Geometry check sheet. Reference: drawing and pictorial views, mm from the part's lowest x, y, z. Round coordinates to 2 decimals unless told otherwise and drop trailing zeros. Loops run counter-clockwise (first coordinate to the right, second up) from the corner with the lowest first, then second, coordinate; pieces in that order, holes last. Notation, with made-up numbers: (-39.5, 17.25) - (8.5, 17.25) arc R14 cw to (8.5, 39.25) - close; hole circle Ø7 at (-35, 8.5). An arc over 180 degrees is marked (long way). Put each result on its own line as item: value. Start each with the question number.
Item 1: Section check B-B, the plane x = 25. Record the cut outline in (y, z).
Item 2: Gauge pin test, flat ends, axial feed: pin 1 Ø5 at (x, y) = (153.5, 10.5) entering from -Z; pin 2 Ø4 at (x, z) = (25, 10) entering from +Y; pin 3 Ø2 at (x, z) = (25, 10) entering from +Y; pin 4 Ø4 at (x, z) = (159, 12) entering from +Y. Record the tip position at first contact, or that the pin passes through.
Item 3: Material ranges on line 1 along X through (y, z) = (2.15, 10); line 2 along Z through (x, y) = (25, 4.2); line 3 along Z through (x, y) = (77.5, 7.5), recorded low to high.
Item 4: Section check C-C, the plane x = 162. Record the cut outline in (y, z).
Item 5: Section check A-A, the plane y = 11.5. Record the cut outline in (x, z).
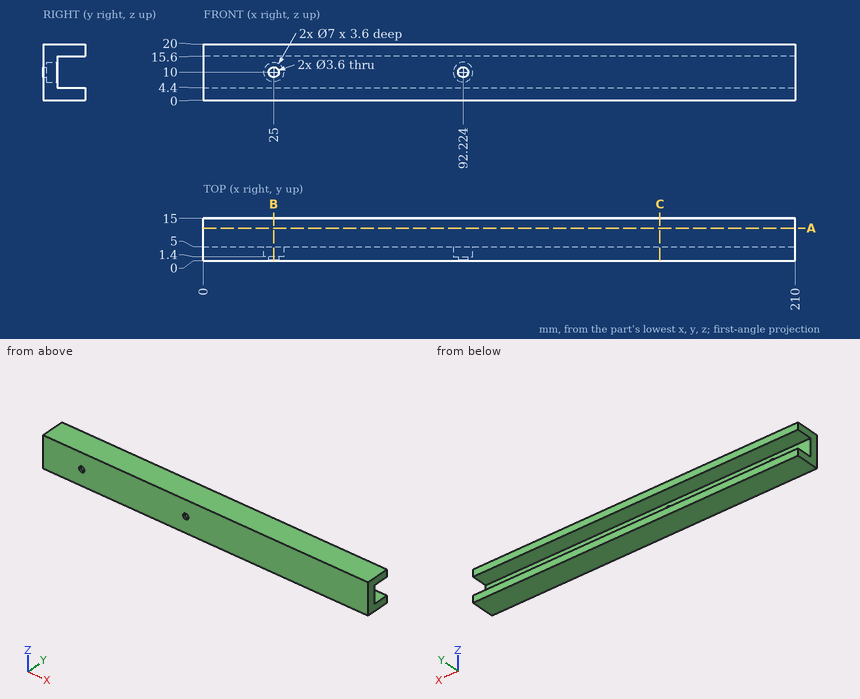
Check result:
1. outline: (0, 0) - (15, 0) - (15, 4.4) - (5, 4.4) - (5, 6.5) - (1.4, 6.5) - (1.4, 8.2) - (0, 8.2) - close; (0, 11.8) - (1.4, 11.8) - (1.4, 13.5) - (5, 13.5) - (5, 15.6) - (15, 15.6) - (15, 20) - (0, 20) - close
2. pin 1: z = 0
2. pin 2: y = 1.4
2. pin 3: through
2. pin 4: y = 5
3. line 1: 0 to 21.5, 28.5 to 88.72, 95.72 to 210
3. line 2: 0 to 6.5, 13.5 to 20
3. line 3: 0 to 4.4, 15.6 to 20
4. outline: (0, 0) - (15, 0) - (15, 4.4) - (5, 4.4) - (5, 15.6) - (15, 15.6) - (15, 20) - (0, 20) - close
5. outline: (0, 0) - (210, 0) - (210, 4.4) - (0, 4.4) - close; (0, 15.6) - (210, 15.6) - (210, 20) - (0, 20) - close
